Here's how the part is built. I have some questions about the finished solid (model axes, mm). Face numbers are marked on the shaded views. A direction names the side the tool comes from. Give positions to 0.01 mm unless a question says otherwise; leave off trailing zeros. Loops run counter-clockwise (first coordinate to the right, second up) from the corner with the lowest first, then second, coordinate; pieces in that order, holes last. Notation, with made-up numbers: (78.25, 0.5) -> (125.25, 0.5) arc R24 ccw to (125.25, 10.5) -> close; hole circle Ø11 at (85, -20). An arc over 180 degrees is marked (long way). Answer in a Markdown table with one row per item. Add a question column.
Item 1: For P1, Ø1.6, axis at y = -13.5, z = -4, coming from the -X side; P2, Ø1.2, axis at x = 0.5, y = -0.5, coming from the -Z side; P3, Ø0.9, axis at y = 0, z = -19, coming from the -X side; P4, Ø9.5, axis at x = -13.5, z = 3, coming from the +Y side, each with a flat end and sliding along its axis, tell me the tip position at first contact or that it passes through.
Item 2: Which directions (+Z, -Z, +X, -X, +Y, -Y) give clear straight access to the entire face, cutting with the end or side of a thin tool? Please do the marked faces 4, 5 and 6.
Item 3: If I drill on line 1 (Z direction, x = -4.5, y = 3.25); line 2 (Y direction, x = -1, z = -19); line 3 (Y direction, x = 1, z = 24.9), over which ranges is the centre line in solid material (lowest first)?
Item 4: If we section it at D-D (z = 0): Write out the boundary of the cut face in (x, y), then the cut area to 4 significant figures.
Item 5: If we section it at A-A (z = -17.5): Write out the boundary of the cut face in (x, y), then the cut area to 4 significant figures.
Item 6: If we section it at C-C (z = -11.5): Write out the boundary of the cut face in (x, y).
Item 7: If we section it at B-B (y = 0): Give the number of separate pieces and of enclosed holes in the cut face, then the cut area to 3 significant figures.
Item 8: We'd pull the mould along Y, two halves only. Please class the marked faces 1, 2 and 3: released by +Y, released by -Y, zero draft, split by the parting line, or undercut.
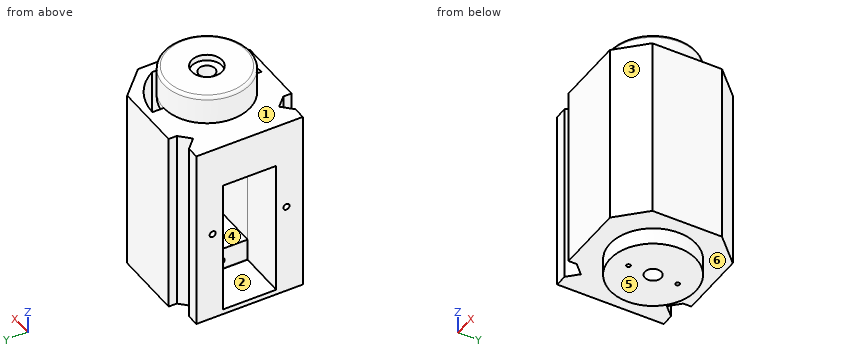
```python
from build123d import *

# Parameters (mm, degrees)
BOSS_EXTRUDE1_DEPTH = 22.5
SKETCH2_R           = 10.5
SKETCH2_R_2         = 2
SKETCH2_R_3         = 0.5
BOSS_EXTRUDE2_DEPTH = 4.1
BOSS_EXTRUDE3_START = 7
SKETCH4_R           = 10.55
SKETCH4_R_2         = 2
BOSS_EXTRUDE3_DEPTH = 7
SKETCH5_R           = 3.75
CUT_EXTRUDE1_DEPTH  = 1.5
CUT_EXTRUDE2_DEPTH  = 15
SKETCH8_W           = 33
SKETCH8_H           = 13
CUT_EXTRUDE4_DEPTH  = 11.75
SKETCH9_W           = 22.9
SKETCH9_H           = 13
CUT_EXTRUDE5_DEPTH  = 17
SKETCH10_R          = 0.75
CUT_EXTRUDE6_DEPTH  = 8
SKETCH11_R          = 0.9
CUT_EXTRUDE7_DEPTH  = 10.75
CUT_EXTRUDE8_DEPTH  = 13
FILLET2_R           = 0.75
SKETCH14_W          = 13.5
SKETCH14_H          = 13
CUT_EXTRUDE9_DEPTH  = 7
FILLET3_R           = 6
SKETCH15_W          = 2
SKETCH15_H          = 20.442632008
CUT_EXTRUDE10_DEPTH = 54.926431367
SKETCH16_W          = 2.396552237
SKETCH16_H          = 13
BOSS_EXTRUDE5_DEPTH = 15
CHAMFER1_SIZE       = 0.35
CHAMFER1_SIZE_2     = 1
SKETCH17_W          = 0.25
SKETCH17_H          = 13
CUT_EXTRUDE11_DEPTH = 11.75


with BuildPart() as part:
    # Sketch1 → Boss-Extrude1 (new, symmetric)
    with BuildSketch(Plane.XY):
        Polygon((8.5, 15), (16, 7.5), (16, -7.5), (8.5, -15), (-8.5, -15), (-8.5, -13), (-11, -10.5), (-13.5, -13), (-16.5, -13), (-16.5, 13), (-13.5, 13), (-11, 10.5), (-8.5, 13), (-8.5, 15), align=None)
    extrude(amount=BOSS_EXTRUDE1_DEPTH, both=True)

    # Sketch2 → Boss-Extrude2 (add)
    with BuildSketch(Plane(origin=(0, 0, -22.5), x_dir=(-1, 0, 0), z_dir=(0, 0, -1))):
        with Locations((-1, 0)):
            Circle(SKETCH2_R)
        with Locations((-1, 0)):
            Circle(SKETCH2_R_2, mode=Mode.SUBTRACT)
        with Locations((-1, 6)):
            Circle(SKETCH2_R_3, mode=Mode.SUBTRACT)
        with Locations((-1, -6)):
            Circle(SKETCH2_R_3, mode=Mode.SUBTRACT)
    extrude(amount=BOSS_EXTRUDE2_DEPTH)

    # Sketch4 → Boss-Extrude3 (add)
    with BuildSketch(Plane.XY.offset(22.5).offset(BOSS_EXTRUDE3_START)):
        with Locations(Location((1, 0, 0), (0, 0, 180))):
            Circle(SKETCH4_R)
        with Locations(Location((1, 0, 0), (0, 0, 180))):
            Circle(SKETCH4_R_2, mode=Mode.SUBTRACT)
    extrude(amount=-BOSS_EXTRUDE3_DEPTH)

    # Sketch5 → Cut-Extrude1 (cut)
    with BuildSketch(Plane.XY.offset(29.5)):
        with Locations((1, 0)):
            Circle(SKETCH5_R)
    extrude(amount=-CUT_EXTRUDE1_DEPTH, mode=Mode.SUBTRACT)

    # Sketch6 → Cut-Extrude2 (cut)
    with BuildSketch(Plane.XY.offset(22.5)):
        with BuildLine():
            Line((1, 13.3), (1, 10.55))
            ThreePointArc((1, 10.55), (11.55, 0), (1, -10.55))
            Line((1, -10.55), (1, -13.3))
            ThreePointArc((1, -13.3), (14.3, 0), (1, 13.3))
        make_face()
    extrude(amount=-CUT_EXTRUDE2_DEPTH, mode=Mode.SUBTRACT)

    # Sketch8 → Cut-Extrude4 (cut)
    with BuildSketch(Plane.ZY.offset(16.5)):
        with Locations((-4.5, 0)):
            Rectangle(SKETCH8_W, SKETCH8_H)
    extrude(amount=-CUT_EXTRUDE4_DEPTH, mode=Mode.SUBTRACT)

    # Sketch9 → Cut-Extrude5 (cut)
    with BuildSketch(Plane.ZY.offset(4.75)):
        with Locations((-4.4, 0)):
            Rectangle(SKETCH9_W, SKETCH9_H)
    extrude(amount=-CUT_EXTRUDE5_DEPTH, mode=Mode.SUBTRACT)

    # Sketch10 → Cut-Extrude6 (cut)
    with BuildSketch(Plane.ZY.offset(16.5)):
        with Locations((0, 9)):
            Circle(SKETCH10_R)
        with Locations((0, -9)):
            Circle(SKETCH10_R)
    extrude(amount=-CUT_EXTRUDE6_DEPTH, mode=Mode.SUBTRACT)

    # Sketch11 → Cut-Extrude7 (cut)
    with BuildSketch(Plane.ZY.offset(4.75)):
        with Locations((-19.05, 0)):
            Circle(SKETCH11_R)
        with Locations((8.75, 0)):
            Circle(SKETCH11_R)
    extrude(amount=-CUT_EXTRUDE7_DEPTH, mode=Mode.SUBTRACT)

    # Sketch12 → Cut-Extrude8 (cut)
    with BuildSketch(Plane.XY.offset(20.5)):
        with BuildLine():
            Line((1, 13.3), (1, -13.3))
            ThreePointArc((1, -13.3), (14.3, 0), (1, 13.3))
        make_face()
    extrude(amount=-CUT_EXTRUDE8_DEPTH, mode=Mode.SUBTRACT)

    # Fillet2
    fillet2_edges = [part.edges().sort_by_distance(p)[0] for p in [
        (11.55, 0, 20.5),
        (11.55, 0, 29.5),
    ]]
    fillet(fillet2_edges, radius=FILLET2_R)

    # Sketch14 → Cut-Extrude9 (cut)
    with BuildSketch(Plane(origin=(0, 0, 7.05), x_dir=(-1, 0, 0), z_dir=(0, 0, -1))):
        with Locations((-5.5, 0)):
            Rectangle(SKETCH14_W, SKETCH14_H)
    extrude(amount=-CUT_EXTRUDE9_DEPTH, mode=Mode.SUBTRACT)

    # Fillet3
    # the kernel refuses this fillet: 6 mm, written as the material it takes off along each edge
    with BuildSketch(Plane(origin=(1, 6.5, 7.5), x_dir=(0, 0, -1), z_dir=(1, 0, 0))) as fillet3_piece_1_section:
        with BuildLine():
            CenterArc((FILLET3_R, FILLET3_R), FILLET3_R, 180, 90)
            Line((0, FILLET3_R), (0, 0))
            Line((0, 0), (FILLET3_R, 0))
        make_face()
    fillet3_piece_1 = extrude(amount=8.309783391, mode=Mode.PRIVATE)
    fillet3_piece_1 = fillet3_piece_1 & Plane(origin=(1, 0, 5.762056744), x_dir=(0, -1, 0), z_dir=(0, 0, 1)) * Cylinder(13.3, 41, mode=Mode.PRIVATE)
    add(fillet3_piece_1, mode=Mode.SUBTRACT)
    with BuildSketch(Plane(origin=(9.309783391, -6.5, 7.5), x_dir=(0, -1, 0), z_dir=(-1, 0, 0))) as fillet3_piece_2_section:
        with BuildLine():
            CenterArc((FILLET3_R, -FILLET3_R), FILLET3_R, 90, 90)
            Line((0, -FILLET3_R), (0, 0))
            Line((0, 0), (FILLET3_R, 0))
        make_face()
    fillet3_piece_2 = extrude(amount=8.309783391, mode=Mode.PRIVATE)
    fillet3_piece_2 = fillet3_piece_2 & Plane(origin=(1, 0, 7.288583483), x_dir=(0, -1, 0), z_dir=(0, 0, 1)) * Cylinder(13.3, 41, mode=Mode.PRIVATE)
    add(fillet3_piece_2, mode=Mode.SUBTRACT)
    with BuildSketch(Plane(origin=(12.25, -6.5, 7.5), x_dir=(0, 0, -1), z_dir=(-1, 0, 0))) as fillet3_piece_3_section:
        with BuildLine():
            CenterArc((FILLET3_R, FILLET3_R), FILLET3_R, 180, 90)
            Line((0, FILLET3_R), (0, 0))
            Line((0, 0), (FILLET3_R, 0))
        make_face()
    fillet3_piece_3 = extrude(amount=2.940216609, mode=Mode.PRIVATE)
    fillet3_piece_3 = fillet3_piece_3 & Plane(origin=(1, 0, 5.940678517), x_dir=(0, -1, 0), z_dir=(0, 0, 1)) * Cylinder(13.3, 30, mode=Mode.PRIVATE)
    add(fillet3_piece_3, mode=Mode.SUBTRACT)
    with BuildSketch(Plane(origin=(9.309783391, 6.5, 7.5), x_dir=(0, 0, -1), z_dir=(1, 0, 0))) as fillet3_piece_4_section:
        with BuildLine():
            CenterArc((FILLET3_R, FILLET3_R), FILLET3_R, 180, 90)
            Line((0, FILLET3_R), (0, 0))
            Line((0, 0), (FILLET3_R, 0))
        make_face()
    fillet3_piece_4 = extrude(amount=2.940216609, mode=Mode.PRIVATE)
    fillet3_piece_4 = fillet3_piece_4 & Plane(origin=(1, 0, 5.940678478), x_dir=(0, -1, 0), z_dir=(0, 0, 1)) * Cylinder(13.3, 30, mode=Mode.PRIVATE)
    add(fillet3_piece_4, mode=Mode.SUBTRACT)

    # Sketch15 → Cut-Extrude10 (cut, through all)
    with BuildSketch(Plane.XY.offset(22.5)):
        with Locations((16, 0)):
            Rectangle(SKETCH15_W, SKETCH15_H)
    extrude(amount=-CUT_EXTRUDE10_DEPTH, mode=Mode.SUBTRACT)

    # Sketch16 → Boss-Extrude5 (add)
    with BuildSketch(Plane.XY.offset(22.5)):
        with Locations((13.801723882, 0)):
            Rectangle(SKETCH16_W, SKETCH16_H)
    extrude(amount=-BOSS_EXTRUDE5_DEPTH)

    # Chamfer1
    # the kernel refuses this chamfer: 1, 0.35 mm, written as the material it takes off along each edge
    with BuildSketch(Plane(origin=(12.25, 6.5, 7.5), x_dir=(0.9946410899892074, 0, 0.10338811394488918), z_dir=(0, -1, 0))) as chamfer1_piece_1:
        Polygon((CHAMFER1_SIZE * 0.994641089989, -CHAMFER1_SIZE * 0.103388113945), (-CHAMFER1_SIZE_2 * 0.103388113945, -CHAMFER1_SIZE_2 * 0.994641089989), (0, 0), align=None)
    extrude(amount=13, mode=Mode.SUBTRACT)
    with BuildSketch(Plane(origin=(12.25, 9.688783911, 7.5), x_dir=(0.9946410899892074, 0, 0.10338811394488918), z_dir=(0, -1, 0))) as chamfer1_piece_2_section:
        Polygon((CHAMFER1_SIZE * 0.994641089989, -CHAMFER1_SIZE * 0.103388113945), (-CHAMFER1_SIZE_2 * 0.103388113945, -CHAMFER1_SIZE_2 * 0.994641089989), (0, 0), align=None)
    chamfer1_piece_2 = extrude(amount=3.188783911, mode=Mode.PRIVATE)
    chamfer1_piece_2 = chamfer1_piece_2 & Plane(origin=(1, 0, 7.126715107), x_dir=(0, -1, 0), z_dir=(0, 0, 1)) * Cylinder(13.3, 11, mode=Mode.PRIVATE)
    add(chamfer1_piece_2, mode=Mode.SUBTRACT)
    with BuildSketch(Plane(origin=(12.25, -9.688783911, 7.5), x_dir=(0.9946410899892074, 0, 0.10338811394488918), z_dir=(0, 1, 0))) as chamfer1_piece_3_section:
        Polygon((CHAMFER1_SIZE * 0.994641089989, CHAMFER1_SIZE * 0.103388113945), (-CHAMFER1_SIZE_2 * 0.103388113945, CHAMFER1_SIZE_2 * 0.994641089989), (0, 0), align=None)
    chamfer1_piece_3 = extrude(amount=3.188783911, mode=Mode.PRIVATE)
    chamfer1_piece_3 = chamfer1_piece_3 & Plane(origin=(1, 0, 7.126715107), x_dir=(0, -1, 0), z_dir=(0, 0, 1)) * Cylinder(13.3, 11, mode=Mode.PRIVATE)
    add(chamfer1_piece_3, mode=Mode.SUBTRACT)

    # Sketch17 → Cut-Extrude11 (cut)
    with BuildSketch(Plane.ZY.offset(16.5)):
        with Locations((-21.125, 0)):
            Rectangle(SKETCH17_W, SKETCH17_H)
    extrude(amount=-CUT_EXTRUDE11_DEPTH, mode=Mode.SUBTRACT)


solid = part.part
```
Recorded:
| question | item | result |
|---|---|---|
| 1 | P1 | stops at x = -16.5 |
| 1 | P2 | stops at z = -22.5 |
| 1 | P3 | stops at x = 6 |
| 1 | P4 | stops at y = 13 |
| 2 | face 4 | -X |
| 2 | face 5 | -Z, +X, -X, +Y, -Y |
| 2 | face 6 | -Z |
| 3 | line 1 | z = -26.6 to -15.85, 7.05 to 29.5 |
| 3 | line 2 | y = -15 to -0.9, 0.9 to 15 |
| 3 | line 3 | y = -10.55 to -2, 2 to 10.55 |
| 4 | outline | (-16.5, -13) -> (-13.5, -13) -> (-11, -10.5) -> (-8.5, -13) -> (-8.5, -15) -> (8.5, -15) -> (15, -8.5) -> (15, 8.5) -> (8.5, 15) -> (-8.5, 15) -> (-8.5, 13) -> (-11, 10.5) -> (-13.5, 13) -> (-16.5, 13) -> (-16.5, 9.75) -> (-8.5, 9.75) -> (-8.5, 8.25) -> (-16.5, 8.25) -> (-16.5, 6.5) -> (12.25, 6.5) -> (12.25, -6.5) -> (-16.5, -6.5) -> (-16.5, -8.25) -> (-8.5, -8.25) -> (-8.5, -9.75) -> (-16.5, -9.75) -> close |
| 4 | area | 460.5 mm^2 |
| 5 | outline | (-16.5, -13) -> (-13.5, -13) -> (-11, -10.5) -> (-8.5, -13) -> (-8.5, -15) -> (8.5, -15) -> (15, -8.5) -> (15, 8.5) -> (8.5, 15) -> (-8.5, 15) -> (-8.5, 13) -> (-11, 10.5) -> (-13.5, 13) -> (-16.5, 13) -> (-16.5, 6.5) -> (-4.75, 6.5) -> (-4.75, -6.5) -> (-16.5, -6.5) -> close |
| 5 | area | 705.5 mm^2 |
| 6 | outline | (-16.5, -13) -> (-13.5, -13) -> (-11, -10.5) -> (-8.5, -13) -> (-8.5, -15) -> (8.5, -15) -> (15, -8.5) -> (15, 8.5) -> (8.5, 15) -> (-8.5, 15) -> (-8.5, 13) -> (-11, 10.5) -> (-13.5, 13) -> (-16.5, 13) -> (-16.5, 6.5) -> (12.25, 6.5) -> (12.25, -6.5) -> (-16.5, -6.5) -> close |
| 7 | separate pieces | 3 |
| 7 | enclosed holes | 0 |
| 7 | area | 622 mm^2 |
| 8 | face 1 | zero draft |
| 8 | face 2 | undercut |
| 8 | face 3 | released by -Y |
